Autodesk Inventor part; units mm, degrees
ref_plane "YZ Plane" through (0, 0, 0) normal (1, 0, 0) x (0, 1, 0)
ref_plane "XZ Plane" through (0, 0, 0) normal (0, 1, 0) x (-1, 0, 0)
ref_plane "XY Plane" through (0, 0, 0) normal (0, 0, 1) x (1, 0, 0)
sketch "Sketch1" plane through (0, 0, 0) normal (1, 0, 0) x (0, 1, 0)
  line L0 (0, 0) -> (40, 0)
  line L1 (40, 0) -> (40, 25)
  line L2 (40, 25) -> (0, 25)
  line L3 (0, 25) -> (0, 0)
  line L4 (35.8, 19.9) -> (28, 19.9)
  line L5 (28, 19.9) -> (28, 5.1)
  line L6 (28, 5.1) -> (35.8, 5.1)
  line L7 (35.8, 5.1) -> (35.8, 19.9)
  dimension "d0" = 40
  dimension "d1" = 25
  dimension "d2" = 14.8
  dimension "d3" = 7.8
  dimension "d4" = 5.1
  dimension "d5" = 28
extrude "Extrusion1" add sketch "Sketch1" along normal blind 11.5
sketch "Sketch2" plane through (0, 0, 25) normal (0, 0, 1) x (1, 0, 0)
  line L0 (0, 0) -> (11.5, 0)
  line L1 (11.5, 40) -> (11.5, 0)
  line L2 (0, 0) -> (11.5, 0)
  line L3 (11.5, 0) -> (11.5, 4)
  line L4 (11.5, 4) -> (0, 4)
  line L5 (0, 4) -> (0, 0)
  dimension "d8" = 4
extrude "Extrusion2" add sketch "Sketch2" along normal blind 3
sketch "Sketch3" plane through (0, 0, 0) normal (0, 0, -1) x (-1, 0, 0)
  line L0 (0, 4) -> (-11.5, 4)
  line L1 (0, 4) -> (0, 0)
  line L2 (-11.5, 4) -> (0, 4)
  line L3 (0, 4) -> (0, 0)
  line L4 (0, 0) -> (-11.5, 0)
  line L5 (-11.5, 0) -> (-11.5, 4)
extrude "Extrusion3" add sketch "Sketch3" along normal blind 5
properties part number "SecondaryBracket"
Verification items for the finished model (mm, model axes). A direction names the side the tool comes from. Give positions to 0.01 mm unless a question says otherwise; leave off trailing zeros. Write each loop counter-clockwise with the first axis right and the second up, starting at its lowest first coordinate (ties: lowest second). Pieces come first, ordered by that corner, then holes. Notation, with made-up numbers: M 14,-4 L 35,-4 A27 ccw 35,17 Z; hole C -1.5,-20.5 d7. An arc over 180 degrees is marked long. One line per question, with ' | ' between items.
1) Set-up check for faces 1 (the flat face through (6, 4, 26)), 2 (the flat face through (6, 22, 0)), 3 (the flat face through (6, 0, 12)), 4 (the flat face through (6, 28, 13)): record each of +Z, -Z, +X, -X, +Y, -Y from which the full face is reachable in a straight line by a thin tool's end or side.
Result:
face 1: +Z, +X, -X, +Y | face 2: -Z, +X, -X, +Y | face 3: +Z, -Z, +X, -X, -Y | face 4: +X, -X
2) Section check D-D on y = 26.5. Enter the section's corners in (x, z).
Result:
outline: M 0,0 L 11.5,0 L 11.5,25 L 0,25 Z
3) Section check A-A on z = 12.5. Enter the section's corners in (x, y), plus the area to 3 significant figures.
Result:
outline: M 0,0 L 11.5,0 L 11.5,28 L 0,28 Z; M 0,35.8 L 11.5,35.8 L 11.5,40 L 0,40 Z | area: 370 mm2
4) Section check B-B on y = 33.5. Enter the section's corners in (x, z), plus the area to 3 significant figures.
Result:
outline: M 0,0 L 11.5,0 L 11.5,5.1 L 0,5.1 Z; M 0,19.9 L 11.5,19.9 L 11.5,25 L 0,25 Z | area: 117 mm2
5) Thickness scan on line 1 along Y through (x, z) = (4.5, 13.5); line 2 along Z through (x, y) = (8, 29); line 3 along Z through (x, y) = (5.5, 27.5). Record the ranges inside material, lowest first. Write a range as [from, to].
Result:
line 1: y = [0, 28], [35.8, 40] | line 2: z = [0, 5.1], [19.9, 25] | line 3: z = [0, 25]
6) Mould release check, pull along Z, two halves, no side actions. Record for faces 5 (the flat face through (6, 22, 25)), 6 (the flat face through (6, 32, 5.1)), 7 (the flat face through (6, 4, -2)): released by +Z, released by -Z, zero draft, split by the parting line, or undercut.
Result:
face 5: released by +Z | face 6: undercut | face 7: zero draft
7) Section check C-C on x = 4. Enter the section's corners in (y, z), plus the area to 3 significant figures.
Result:
outline: M 0,-5 L 4,-5 L 4,0 L 40,0 L 40,25 L 4,25 L 4,28 L 0,28 Z; hole M 28,5.1 L 35.8,5.1 L 35.8,19.9 L 28,19.9 Z | area: 917 mm2
8) Gauge pin test, flat ends, axial feed: pin 1 Ø1.5 at (x, z) = (4.5, 4) entering from -Y; pin 2 Ø6 at (x, y) = (4.5, 28.5) entering from -Z; pin 3 Ø4 at (x, y) = (6.5, 31) entering from +Z; pin 4 Ø2.5 at (x, z) = (7.5, -3) entering from +Y. Record the tip position at first contact, or that the pin passes through.
Result:
pin 1: stops at y = 0 | pin 2: stops at z = 0 | pin 3: stops at z = 25 | pin 4: stops at y = 4
